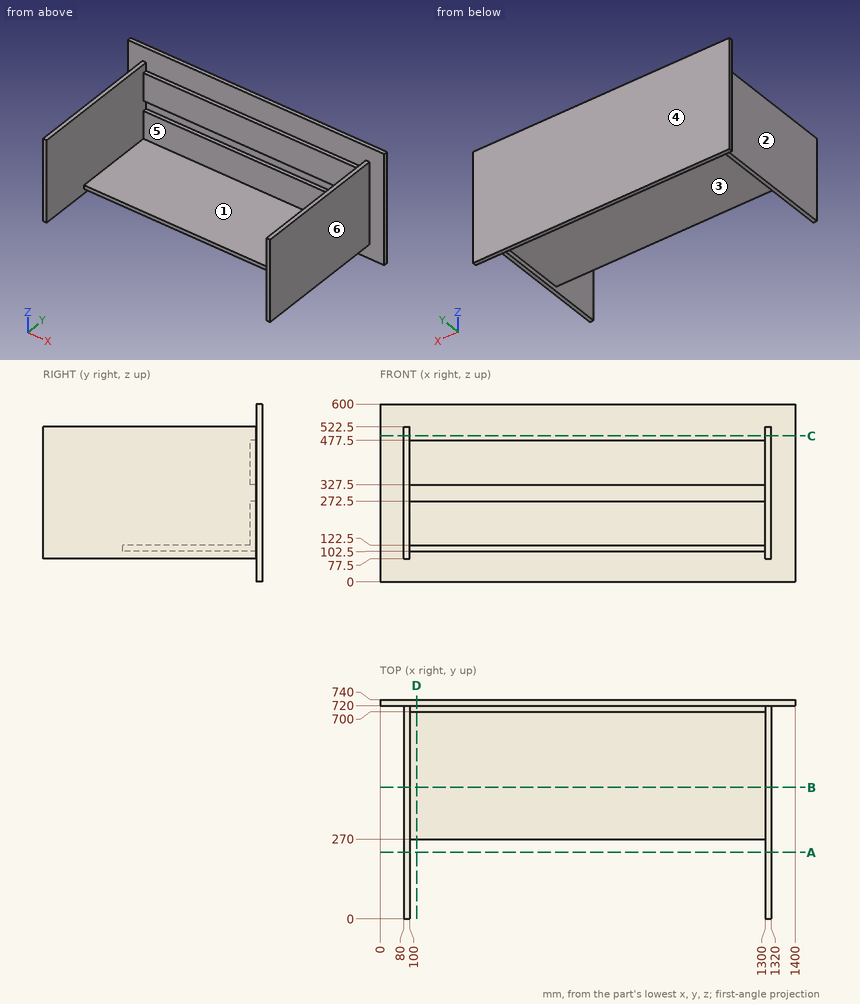
Could you check a few things on this drawing? It's one solid part, dimensions in mm from its lowest x, y, z. A direction names the side the tool comes from. Coordinates: 2 decimals unless noted, no trailing zeros. Order: outer loops, then holes, each group sorted by start corner. A loop starts at its lowest first (then second) coordinate and runs counter-clockwise, first axis right, second up. Notation, with made-up numbers: M 9,-31 L 28,-31 A34 cw 28,-1 Z; hole C 86.5,-5.75 d5. An arc over 180 degrees is marked long. Use a Markdown table: item, result. Add a question column.
Q1. I want a section at B-B on y = 444.5. List the corners of the cut face in (x, z) for me, then the cut area to 3 significant figures.
Q2. I want a section at A-A on y = 224.5. List the corners of the cut face in (x, z) for me, then the cut area to 3 significant figures.
Q3. I want a section at C-C on z = 492. List the corners of the cut face in (x, y) for me.
Q4. I'm going to push flat-ended pins straight in: pin 1 (16 mm diameter, centred on x = 1309, y = 204, fed in from +Z); pin 2 (10 mm diameter, centred on x = 407, y = 706.5, fed in from -Z); pin 3 (3 mm diameter, centred on x = 469, y = 583.5, fed in from +Z). Where does each tip first touch, or does it pass through?
Q5. I want a section at D-D on x = 123. List the corners of the cut face in (y, z) for me.
Q6. We'd pull the mould along X, two halves only. Please class the marked faces 4, 5 and 6: pulls with the +X half, pulls with the -X half, needs draft (parallel to the pull), parting line crosses it, or undercut.
Q7. If I drill on L1, parallel to X at y = 419.5, z = 361.5; L2, parallel to Y at x = 1069, z = 221.5; L3, parallel to Z at x = 1217, y = 660.5, over which ranges is the centre line in solid material (lowest first)?
Q8. Which directions (+Z, -Z, +X, -X, +Y, -Y) give clear straight access to the entire face, cutting with the end or side of a thin tool? Please do the marked faces 1, 2 and 3.
Checked values:
| question | item | result |
|---|---|---|
| 1 | outline | M 80,77.5 L 100,77.5 L 100,102.5 L 1300,102.5 L 1300,77.5 L 1320,77.5 L 1320,522.5 L 1300,522.5 L 1300,122.5 L 100,122.5 L 100,522.5 L 80,522.5 Z |
| 1 | area | 41,800 mm² |
| 2 | outline | M 80,77.5 L 100,77.5 L 100,522.5 L 80,522.5 Z; M 1300,77.5 L 1320,77.5 L 1320,522.5 L 1300,522.5 Z |
| 2 | area | 17,800 mm² |
| 3 | outline | M 0,720 L 80,720 L 80,0 L 100,0 L 100,720 L 1300,720 L 1300,0 L 1320,0 L 1320,720 L 1400,720 L 1400,740 L 0,740 Z |
| 4 | pin 1 | z = 522.5 |
| 4 | pin 2 | z = 102.5 |
| 4 | pin 3 | z = 122.5 |
| 5 | outline | M 270,102.5 L 720,102.5 L 720,0 L 740,0 L 740,600 L 720,600 L 720,477.5 L 700,477.5 L 700,327.5 L 720,327.5 L 720,272.5 L 700,272.5 L 700,122.5 L 270,122.5 Z |
| 6 | face 4 | needs draft |
| 6 | face 5 | undercut |
| 6 | face 6 | pulls with the +X half |
| 7 | L1 | 80 to 100, 1300 to 1320 |
| 7 | L2 | 700 to 740 |
| 7 | L3 | 102.5 to 122.5 |
| 8 | face 1 | +Z, -Y |
| 8 | face 2 | +Z, -Z, -X, -Y |
| 8 | face 3 | -Z, -Y |
